```python
from build123d import *

# Parameters (mm, degrees)
SKETCH1_W           = 76.2
SKETCH1_H           = 101.6
BOSS_EXTRUDE1_DEPTH = 12.7
SKETCH2_W           = 38.1
SKETCH2_H           = 20.6502
CUT_EXTRUDE1_DEPTH  = 4.7498
SKETCH3_R           = 3.81
CUT_EXTRUDE2_DEPTH  = 6.35


with BuildPart() as part:
    # Sketch1 → Boss-Extrude1 (new body)
    with BuildSketch(Plane(origin=(0, 0, 0), x_dir=(1, 0, 0), z_dir=(0, 1, 0))):
        Rectangle(SKETCH1_W, SKETCH1_H)
    extrude(amount=BOSS_EXTRUDE1_DEPTH)

    # Sketch2 → Cut-Extrude1 (cut)
    with BuildSketch(Plane.XZ):
        with Locations((0, 40.4749)):
            Rectangle(SKETCH2_W, SKETCH2_H)
    extrude(amount=-CUT_EXTRUDE1_DEPTH, mode=Mode.SUBTRACT)

    # Sketch3 → Cut-Extrude2 (cut)
    with BuildSketch(Plane(origin=(0, 0, -50.8), x_dir=(-1, 0, 0), z_dir=(0, 0, -1))):
        with Locations((0, 6.35)):
            Circle(SKETCH3_R)
    extrude(amount=-CUT_EXTRUDE2_DEPTH, mode=Mode.SUBTRACT)


solid = part.part
```
Check sheet for the modelled part. Datum: model origin and axes. Units: mm. A direction names the side the tool comes from. Give positions to 0.01 mm unless a question says otherwise; leave off trailing zeros. Write each loop counter-clockwise with the first axis right and the second up, starting at its lowest first coordinate (ties: lowest second). Pieces come first, ordered by that corner, then holes. Notation, with made-up numbers: (45, -30) -> (56, -30) arc R22 ccw to (56, -16) -> close; hole circle Ø9 at (54, -11.75). An arc over 180 degrees is marked (long way). Use CSV: the item, a comma, the result in double quotes. Start each with the question number.
Q1. Cross-section at B-B on x = 13.5. Enter the section's corners in (y, z), and give its area (3 significant figures).
Q2. Tool access check on faces 4 (the flat face through (0, 6, -44.45)), 5 (the flat face through (19.05, 2, 40)), 6 (the flat face through (-0.5, 10.5, -50.8)). Record the directions out of +Z, -Z, +X, -X, +Y, -Y that give a thin tool (end or side, any length) a straight path to the whole face; none if there is none.
Q3. Scan lines: line 1 along Y through (x, z) = (0, -48.5); line 2 along Z through (x, y) = (0, 1.75); line 3 along Z through (x, y) = (1, 9.5). Record each from-to range of solid material in increasing order.
Q4. Cross-section at A-A on x = 0. Enter the section's corners in (y, z), and give its area (3 significant figures).
Q5. Release check for a two-part mould opening along Y. For faces 1 (the flat face through (-1, 8, 50.8)), 2 (the flat face through (-1, 12.7, -1)), 3 (the cylindrical face through (0.496, 10.128, -47.669)) record: +Y half, -Y half, draft (parallel to the pull), parting line (faces both ways), or undercut.
Q6. Depth check by flat-ended pin: P1, Ø6, axis at x = 0, y = 6.35, coming from the -Z side; P2, Ø4, axis at x = 1, y = 2, coming from the +Z side; P3, Ø10.5, axis at x = -0.5, z = 42, coming from the -Y side. Enter the tip coordinate at first touch or a pass-through.
Working result:
1,outline,"(0, -50.8) -> (12.7, -50.8) -> (12.7, 50.8) -> (4.75, 50.8) -> (4.75, 30.15) -> (0, 30.15) -> close"
1,area,"1,190 mm^2"
2,face 4,"-Z"
2,face 5,"+Z, -Y"
2,face 6,"-Z, +X, -X, +Y, -Y"
3,line 1,"y = 0 to 2.54, 10.16 to 12.7"
3,line 2,"z = -50.8 to 30.15"
3,line 3,"z = -44.45 to 50.8"
4,outline,"(0, -50.8) -> (2.54, -50.8) -> (2.54, -44.45) -> (10.16, -44.45) -> (10.16, -50.8) -> (12.7, -50.8) -> (12.7, 50.8) -> (4.75, 50.8) -> (4.75, 30.15) -> (0, 30.15) -> close"
4,area,"1,140 mm^2"
5,face 1,"draft"
5,face 2,"+Y half"
5,face 3,"undercut"
6,P1,"stops at z = -44.45"
6,P2,"stops at z = 30.15"
6,P3,"stops at y = 4.75"
